from build123d import *

# Parameters (mm, degrees)
SKETCH1_R               = 2.2479
SKETCH1_R_2             = 3.81
BOSS_EXTRUDE1_DEPTH     = 6.35
CUT_EXTRUDE1_DEPTH      = 217.831812703
CUT_EXTRUDE1_DEPTH_BACK = 217.831812703
SKETCH3_W               = 3.81
SKETCH3_H               = 15.875
CUT_EXTRUDE2_DEPTH      = 217.831812703
FILLET1_R               = 1.524


with BuildPart() as part:
    # Sketch1 → Boss-Extrude1 (new body)
    with BuildSketch(Plane(origin=(0, 0, 0), x_dir=(1, 0, 0), z_dir=(0, 1, 0))):
        with BuildLine():
            Line((-180.975, 114.3), (180.975, 114.3))
            ThreePointArc((180.975, 114.3), (183.22006403, 113.37006403), (184.15, 111.125))
            Line((184.15, 111.125), (184.15, -111.125))
            ThreePointArc((184.15, -111.125), (183.22006403, -113.37006403), (180.975, -114.3))
            Line((180.975, -114.3), (-180.975, -114.3))
            ThreePointArc((-180.975, -114.3), (-183.22006403, -113.37006403), (-184.15, -111.125))
            Line((-184.15, -111.125), (-184.15, 111.125))
            ThreePointArc((-184.15, 111.125), (-183.22006403, 113.37006403), (-180.975, 114.3))
        make_face()
        with Locations(Location((-149.225, -104.775, 0), (0, 0, 270))):
            Circle(SKETCH1_R, mode=Mode.SUBTRACT)
        with Locations(Location((-55.033333333, -104.775, 0), (0, 0, 270))):
            Circle(SKETCH1_R, mode=Mode.SUBTRACT)
        with Locations(Location((55.033333333, -104.775, 0), (0, 0, 270))):
            Circle(SKETCH1_R, mode=Mode.SUBTRACT)
        with Locations(Location((165.1, -104.775, 0), (0, 0, 270))):
            Circle(SKETCH1_R, mode=Mode.SUBTRACT)
        with Locations(Location((165.1, 104.775, 0), (0, 0, 270))):
            Circle(SKETCH1_R, mode=Mode.SUBTRACT)
        with Locations(Location((55.033333333, 104.775, 0), (0, 0, 270))):
            Circle(SKETCH1_R, mode=Mode.SUBTRACT)
        with Locations(Location((-55.033333333, 104.775, 0), (0, 0, 270))):
            Circle(SKETCH1_R, mode=Mode.SUBTRACT)
        with Locations(Location((-149.225, 104.775, 0), (0, 0, 270))):
            Circle(SKETCH1_R, mode=Mode.SUBTRACT)
        with Locations(Location((-55.033333333, 0, 0), (0, 0, 270))):
            Circle(SKETCH1_R, mode=Mode.SUBTRACT)
        with Locations(Location((55.033333333, 0, 0), (0, 0, 270))):
            Circle(SKETCH1_R, mode=Mode.SUBTRACT)
        with Locations(Location((-55.0291, 80.01, 0), (0, 0, 270))):
            Circle(SKETCH1_R_2, mode=Mode.SUBTRACT)
        with Locations(Location((-55.0291, -80.01, 0), (0, 0, 270))):
            Circle(SKETCH1_R_2, mode=Mode.SUBTRACT)
        with Locations(Location((55.0291, -80.01, 0), (0, 0, 270))):
            Circle(SKETCH1_R_2, mode=Mode.SUBTRACT)
        with Locations(Location((55.0291, 80.01, 0), (0, 0, 270))):
            Circle(SKETCH1_R_2, mode=Mode.SUBTRACT)
        with Locations(Location((165.1, 0, 0), (0, 0, 270))):
            Circle(SKETCH1_R, mode=Mode.SUBTRACT)
        with Locations(Location((-171.45, 0, 0), (0, 0, 270))):
            Circle(SKETCH1_R, mode=Mode.SUBTRACT)
        with BuildLine():
            Line((-24.3078, -3.1623), (24.3078, -3.1623))
            ThreePointArc((24.3078, -3.1623), (55.879209158, -53.5178), (24.3078, -103.8733))
            Line((24.3078, -103.8733), (-24.3078, -103.8733))
            ThreePointArc((-24.3078, -103.8733), (-55.879209158, -53.5178), (-24.3078, -3.1623))
        make_face(mode=Mode.SUBTRACT)
        with BuildLine():
            Line((95.136490842, -3.1623), (143.752090842, -3.1623))
            ThreePointArc((143.752090842, -3.1623), (175.3235, -53.5178), (143.752090842, -103.8733))
            Line((143.752090842, -103.8733), (95.136490842, -103.8733))
            ThreePointArc((95.136490842, -103.8733), (63.565081684, -53.5178), (95.136490842, -3.1623))
        make_face(mode=Mode.SUBTRACT)
        with BuildLine():
            Line((-143.752090842, -3.1623), (-95.136490842, -3.1623))
            ThreePointArc((-95.136490842, -3.1623), (-63.565081684, -53.5178), (-95.136490842, -103.8733))
            Line((-95.136490842, -103.8733), (-143.752090842, -103.8733))
            ThreePointArc((-143.752090842, -103.8733), (-175.3235, -53.5178), (-143.752090842, -3.1623))
        make_face(mode=Mode.SUBTRACT)
        with BuildLine():
            Line((-24.3078, 103.8733), (24.3078, 103.8733))
            ThreePointArc((24.3078, 103.8733), (55.879209158, 53.5178), (24.3078, 3.1623))
            Line((24.3078, 3.1623), (-24.3078, 3.1623))
            ThreePointArc((-24.3078, 3.1623), (-55.879209158, 53.5178), (-24.3078, 103.8733))
        make_face(mode=Mode.SUBTRACT)
        with BuildLine():
            Line((-143.752090842, 103.8733), (-95.136490842, 103.8733))
            ThreePointArc((-95.136490842, 103.8733), (-63.565081684, 53.5178), (-95.136490842, 3.1623))
            Line((-95.136490842, 3.1623), (-143.752090842, 3.1623))
            ThreePointArc((-143.752090842, 3.1623), (-175.3235, 53.5178), (-143.752090842, 103.8733))
        make_face(mode=Mode.SUBTRACT)
        with BuildLine():
            Line((95.136490842, 103.8733), (143.752090842, 103.8733))
            ThreePointArc((143.752090842, 103.8733), (175.3235, 53.5178), (143.752090842, 3.1623))
            Line((143.752090842, 3.1623), (95.136490842, 3.1623))
            ThreePointArc((95.136490842, 3.1623), (63.565081684, 53.5178), (95.136490842, 103.8733))
        make_face(mode=Mode.SUBTRACT)
    extrude(amount=BOSS_EXTRUDE1_DEPTH)

    # Sketch2 → Cut-Extrude1 (cut, two sides: drawn at the far end of the back side and taken through both)
    with BuildSketch(Plane(origin=(0, 6.35, 0), x_dir=(1, 0, 0), z_dir=(0, 1, 0)).offset(-CUT_EXTRUDE1_DEPTH_BACK)):
        with BuildLine():
            Line((184.15, 25.4), (177.8, 25.4))
            ThreePointArc((177.8, 25.4), (173.309871939, 23.540128061), (171.45, 19.05))
            Line((171.45, 19.05), (171.45, -19.05))
            ThreePointArc((171.45, -19.05), (173.309871939, -23.540128061), (177.8, -25.4))
            Line((177.8, -25.4), (184.15, -25.4))
            Line((184.15, -25.4), (184.15, 25.4))
        make_face()
    extrude(amount=CUT_EXTRUDE1_DEPTH + CUT_EXTRUDE1_DEPTH_BACK, mode=Mode.SUBTRACT)

    # Sketch3 → Cut-Extrude2 (cut, through all)
    with BuildSketch(Plane(origin=(0, 6.35, 0), x_dir=(1, 0, 0), z_dir=(0, 1, 0))):
        with Locations((-182.245, 45.72)):
            Rectangle(SKETCH3_W, SKETCH3_H)
        with Locations((-182.245, -45.72)):
            Rectangle(SKETCH3_W, SKETCH3_H)
    extrude(amount=-CUT_EXTRUDE2_DEPTH, mode=Mode.SUBTRACT)

    # Fillet1
    fillet1_edges = [part.edges().sort_by_distance(p)[0] for p in [
        (184.15, 3.175, -25.4),
        (184.15, 3.175, 25.4),
        (-184.15, 3.175, -37.7825),
        (-184.15, 3.175, -53.6575),
        (-180.34, 3.175, -53.6575),
        (-180.34, 3.175, -37.7825),
        (-184.15, 3.175, 53.6575),
        (-184.15, 3.175, 37.7825),
        (-180.34, 3.175, 37.7825),
        (-180.34, 3.175, 53.6575),
    ]]
    fillet(fillet1_edges, radius=FILLET1_R)


solid = part.part
Could you check a few things on this model? Use its own coordinates, in mm. A direction names the side the tool comes from. Coordinates: 2 decimals unless noted, no trailing zeros. Order: outer loops, then holes, each group sorted by start corner. A loop starts at its lowest first (then second) coordinate and runs counter-clockwise, first axis right, second up. Notation, with made-up numbers: (14, 30.25) -> (72, 30.25) arc R30 ccw to (72, 66.25) -> close; hole circle Ø2 at (17.5, -25). An arc over 180 degrees is marked (long way). One line per item, written item: value. Start each with the question number.
1) I'm going to push flat-ended pins straight in: pin 1 (0.6 mm diameter, centred on x = -182.5, y = 2, fed in from +Z); pin 2 (0.6 mm diameter, centred on x = -182.5, y = 4.5, fed in from -Z); pin 3 (0.8 mm diameter, centred on x = -182, y = 4, fed in from +Z). Where does each tip first touch, or does it pass through?
2) Which directions (+Z, -Z, +X, -X, +Y, -Y) give clear straight access to the entire face, cutting with the end or side of a thin tool? Please do faces 3 (the cylindrical face through (-55.872, 3.131, 54.395)), 4 (the flat face through (1, 6.35, -1)).
3) If I drill on L1, parallel to Z at x = 138.5, y = 1.5; L2, parallel to X at y = 4, z = 0; L3, parallel to X at y = 1.25, z = 49.5, over which ranges is the centre line in solid material (lowest first)? Write a range as [from, to].
4) Imagine slicing it at A-A on z = -93. List the corners of the cut face in (x, y) for me.
5) We'd pull the mould along X, two halves only. Please class faces 1 (the flat face through (1, 0, -1)), 2 (the cylindrical face through (63.57, 3.13, -52.64)): +X half, -X half, draft (parallel to the pull), parting line (faces both ways), or undercut.
6) Imagine slicing it at D-D on x = -156. List the corners of the cut face in (y, z) for me.
7) Imagine slicing it at B-B on x = -14. List the corners of the cut face in (y, z) for me.
8) Imagine slicing it at C-C on z = 80.01. List the corners of the cut face in (x, y) for me, plus the area to 3 significant figures.
Answer list:
1. pin 1: stops at z = 114.05
1. pin 2: stops at z = -114.05
1. pin 3: stops at z = 114.24
2. face 3: +Y, -Y
2. face 4: +Z, -Z, +X, -X, +Y
3. L1: z = [-114.3, -103.87], [-3.16, 3.16], [103.87, 114.3]
3. L2: x = [-184.15, -173.7], [-169.2, -57.28], [-52.79, 52.79], [57.28, 162.85], [167.35, 171.45]
3. L3: x = [-180.34, -175.18], [-63.71, -55.73], [55.73, 63.71], [175.18, 184.15]
4. outline: (-184.15, 0) -> (-159.01, 0) -> (-159.01, 6.35) -> (-184.15, 6.35) -> close; (-79.87, 0) -> (-39.57, 0) -> (-39.57, 6.35) -> (-79.87, 6.35) -> close; (39.57, 0) -> (79.87, 0) -> (79.87, 6.35) -> (39.57, 6.35) -> close; (159.01, 0) -> (184.15, 0) -> (184.15, 6.35) -> (159.01, 6.35) -> close
5. face 1: draft
5. face 2: undercut
6. outline: (0, -114.3) -> (6.35, -114.3) -> (6.35, -95.81) -> (0, -95.81) -> close; (0, -11.23) -> (6.35, -11.23) -> (6.35, 11.23) -> (0, 11.23) -> close; (0, 95.81) -> (6.35, 95.81) -> (6.35, 114.3) -> (0, 114.3) -> close
7. outline: (0, -114.3) -> (6.35, -114.3) -> (6.35, -103.87) -> (0, -103.87) -> close; (0, -3.16) -> (6.35, -3.16) -> (6.35, 3.16) -> (0, 3.16) -> close; (0, 103.87) -> (6.35, 103.87) -> (6.35, 114.3) -> (0, 114.3) -> close
8. outline: (-184.15, 0) -> (-168.65, 0) -> (-168.65, 6.35) -> (-184.15, 6.35) -> close; (-70.24, 0) -> (-58.84, 0) -> (-58.84, 6.35) -> (-70.24, 6.35) -> close; (-51.22, 0) -> (-49.21, 0) -> (-49.21, 6.35) -> (-51.22, 6.35) -> close; (49.21, 0) -> (51.22, 0) -> (51.22, 6.35) -> (49.21, 6.35) -> close; (58.84, 0) -> (70.24, 0) -> (70.24, 6.35) -> (58.84, 6.35) -> close; (168.65, 0) -> (184.15, 0) -> (184.15, 6.35) -> (168.65, 6.35) -> close
8. area: 367 mm2
